Read the model definition and answer for the solid it produces. Units are mm, in the model's axes. Face numbers are marked on the shaded views. A direction names the side the tool comes from. Give positions to 0.01 mm unless a question says otherwise; leave off trailing zeros. Loops run counter-clockwise (first coordinate to the right, second up) from the corner with the lowest first, then second, coordinate; pieces in that order, holes last. Notation, with made-up numbers: (84.5, -15) - (109.5, -15) arc R28 ccw to (109.5, 9) - close; hole circle Ø2 at (46.5, 88). An arc over 180 degrees is marked (long way). Write each question's results on one line, items separated by ' | '. Start each with the question number.
Q1. For the marked faces 1, 2, 3, 4 and 5, determine the directions among +Z, -Z, +X, -X, +Y, -Y from which every point of the face is accessible in a straight line to the end or side of a thin tool.
Q2. Given pin 1 (0.6 mm diameter, centred on y = 22, z = -0.5, fed in from -X); pin 2 (3.5 mm diameter, centred on x = -24.02, y = 15.47, fed in from +Z) (3 decimals); pin 3 (7 mm diameter, centred on x = -15, y = 12, fed in from -Z), each flat-ended and moving along its own axis, determine where each tip first touches the part or whether it passes through.
Q3. The part is cut by section D-D, the plane z = 1.5. Write down the section's boundary in (x, y).
Q4. Find the intervals of material crossed by line 1 (Z direction, x = -12.25, y = 16); line 2 (Z direction, x = -6.25, y = 17.5) (3 decimals); line 3 (Y direction, x = -16.25, z = 3.25), in increasing order. Write a range as from..to.
Q5. The part is cut by section C-C, the plane x = -2.25. Write down the section's boundary in (y, z) (3 decimals), plus the area to 3 significant figures.
Q6. The part is cut by section B-B, the plane y = 21. Write down the section's boundary in (x, z) (3 decimals), plus the area to 3 significant figures.
Q7. The part is cut by section A-A, the plane y = 15. Write down the section's boundary in (x, z) (3 decimals).
```python
from build123d import *

# Parameters (mm, degrees)
SKETCH1_W           = 25.0444
SKETCH1_H           = 23.9522
BOSS_EXTRUDE1_DEPTH = 3.175
SKETCH2_R           = 1.0922
CUT_EXTRUDE1_DEPTH  = 3.175
SKETCH3_W           = 8.0518
SKETCH3_H           = 8.0518
BOSS_EXTRUDE2_DEPTH = 3.937
SKETCH4_W           = 20.8788
SKETCH4_H           = 5.5372
BOSS_EXTRUDE3_DEPTH = 0.5588
SKETCH5_W           = 15.9258
SKETCH5_H           = 0.191961024
BOSS_EXTRUDE4_DEPTH = 7.239


with BuildPart() as part:
    # Sketch1 → Boss-Extrude1 (new body)
    with BuildSketch(Plane.XY):
        with Locations((-13.304877678, 12.887280749)):
            Rectangle(SKETCH1_W, SKETCH1_H)
    extrude(amount=BOSS_EXTRUDE1_DEPTH)

    # Sketch2 → Cut-Extrude1 (cut)
    with BuildSketch(Plane.XY.offset(3.175)):
        with Locations((-2.586077678, 2.714580749)):
            Circle(SKETCH2_R)
        with Locations((-2.586077678, 15.465380749)):
            Circle(SKETCH2_R)
        with Locations((-24.023677678, 2.714580749)):
            Circle(SKETCH2_R)
        with Locations((-24.023677678, 15.465380749)):
            Circle(SKETCH2_R)
    extrude(amount=-CUT_EXTRUDE1_DEPTH, mode=Mode.SUBTRACT)

    # Sketch3 → Boss-Extrude2 (add)
    with BuildSketch(Plane.XY.offset(3.175)):
        with Locations((-13.304877678, 15.046280749)):
            Rectangle(SKETCH3_W, SKETCH3_H)
    extrude(amount=BOSS_EXTRUDE2_DEPTH)

    # Sketch4 → Boss-Extrude3 (add)
    with BuildSketch(Plane(origin=(0, 0, 0), x_dir=(-1, 0, 0), z_dir=(0, 0, -1))):
        with Locations((13.304877678, 22.094780749)):
            Rectangle(SKETCH4_W, SKETCH4_H)
    extrude(amount=BOSS_EXTRUDE3_DEPTH)

    # Sketch5 → Boss-Extrude4 (add)
    with BuildSketch(Plane(origin=(0, 24.863380749, 0), x_dir=(1, 0, 0), z_dir=(0, 1, 0))):
        with Locations((-13.304877678, -0.172180512)):
            Rectangle(SKETCH5_W, SKETCH5_H)
    extrude(amount=BOSS_EXTRUDE4_DEPTH)


solid = part.part
```
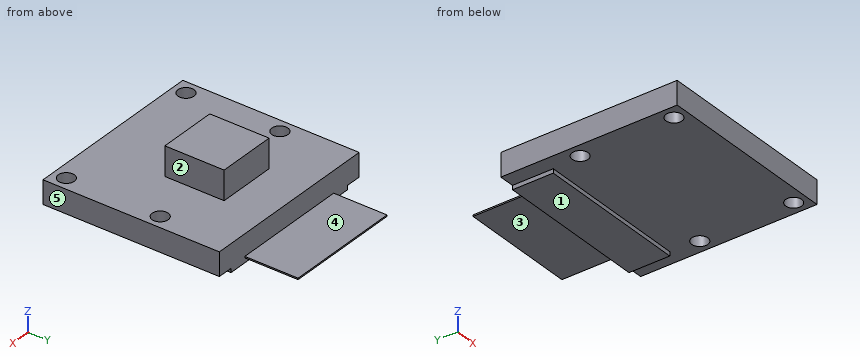
Check sheet entries:
1) face 1: -Z, +X, -X, +Y, -Y | face 2: +Z, +X, +Y, -Y | face 3: -Z, +X, -X, +Y | face 4: +Z, +X, -X, +Y | face 5: +Z, -Z, +X, +Y, -Y
2) pin 1: stops at x = -23.74 | pin 2: stops at z = 3.175 | pin 3: stops at z = 0
3) outline: (-25.83, 0.91) - (-0.78, 0.91) - (-0.78, 24.86) - (-25.83, 24.86) - close; hole circle Ø2.18 at (-24.02, 2.71); hole circle Ø2.18 at (-24.02, 15.47); hole circle Ø2.18 at (-2.59, 2.71); hole circle Ø2.18 at (-2.59, 15.47)
4) line 1: z = 0..7.11 | line 2: z = 0..3.175 | line 3: y = 11.02..19.07
5) outline: (0.911, 0) - (1.675, 0) - (1.675, 3.175) - (0.911, 3.175) - close; (3.754, 0) - (14.426, 0) - (14.426, 3.175) - (3.754, 3.175) - close; (16.505, 0) - (24.863, 0) - (24.863, 3.175) - (16.505, 3.175) - close | area: 62.9 mm^2
6) outline: (-25.827, 0) - (-23.744, 0) - (-23.744, -0.559) - (-2.865, -0.559) - (-2.865, 0) - (-0.783, 0) - (-0.783, 3.175) - (-25.827, 3.175) - close | area: 91.2 mm^2
7) outline: (-25.827, 0) - (-25.012, 0) - (-25.012, 3.175) - (-25.827, 3.175) - close; (-23.036, 0) - (-3.574, 0) - (-3.574, 3.175) - (-9.279, 3.175) - (-9.279, 7.112) - (-17.331, 7.112) - (-17.331, 3.175) - (-23.036, 3.175) - close; (-1.598, 0) - (-0.783, 0) - (-0.783, 3.175) - (-1.598, 3.175) - close
